from build123d import *

# Parameters (mm, degrees)
PAD002_DEPTH            = 5
SKETCH015_R             = 35
SKETCH015_R_2           = 1.6
POCKET005_DEPTH         = 5.001
SKETCH013_R             = 3.5
SKETCH013_R_2           = 1.7
POCKET004_DEPTH         = 5.001
SKETCH025_W             = 47
SKETCH025_H             = 51
POCKET027_DEPTH         = 2.5
BODY002_PLACEMENT_ANGLE = 180


with BuildPart() as part:
    # Sketch014 → Pad002 (new body)
    with BuildSketch(Plane.XY):
        with BuildLine():
            Line((0, 67.42), (0, -55.65))
            Line((0, -55.65), (-117.94, -55.65))
            ThreePointArc((-127.64, -49.11), (-122.947197, -52.613151), (-117.94, -55.65))
            ThreePointArc((-146.95, -26.77), (-138.520798, -38.999541), (-127.64, -49.11))
            ThreePointArc((-148.54, 6.09), (-150.980867, -10.496574), (-146.95, -26.77))
            ThreePointArc((-134.5, 26.2), (-142.831473, 17.060618), (-148.54, 6.09))
            ThreePointArc((-94.13, 48.54), (-115.023795, 38.650843), (-134.5, 26.2))
            ThreePointArc((0, 67.42), (-48.036997, 62.826084), (-94.13, 48.54))
        make_face()
    extrude(amount=PAD002_DEPTH)

    # Sketch015 (on Face10 of Pad002) → Pocket005 (cut, through all)
    with BuildSketch(Plane.XY.offset(5)):
        with Locations((-90.05, -4.36)):
            Circle(SKETCH015_R)
        with Locations((-119.571708, 25.161708)):
            Circle(SKETCH015_R_2)
        with Locations((-60.528292, 25.161708)):
            Circle(SKETCH015_R_2)
        with Locations((-60.528292, -33.881708)):
            Circle(SKETCH015_R_2)
        with Locations((-119.571708, -33.881708)):
            Circle(SKETCH015_R_2)
    extrude(amount=-POCKET005_DEPTH, mode=Mode.SUBTRACT)

    # Sketch013 (on Face5 of Pocket005) → Pocket004 (cut, through all)
    with BuildSketch(Plane.XY.offset(5)):
        with Locations((-30, -40)):
            Circle(SKETCH013_R)
        with Locations((-43.55, 21.8)):
            Circle(SKETCH013_R_2)
        with Locations((-43.55, -21.8)):
            Circle(SKETCH013_R_2)
        Polygon((0, 25.5), (-38.85, 25.5), (-38.85, 18.5), (-46.75, 18.5), (-46.75, -18.5), (-38.85, -18.5), (-38.85, -25.5), (0, -25.5), align=None)
    extrude(amount=-POCKET004_DEPTH, mode=Mode.SUBTRACT)

    # Sketch025 → Pocket027 (cut)
    with BuildSketch(Plane.XY):
        with Locations((-23.5, 0)):
            Rectangle(SKETCH025_W, SKETCH025_H)
    extrude(amount=POCKET027_DEPTH, mode=Mode.SUBTRACT)


with BuildPart() as part_1:
    # Body002 placement: moved
    add(part.part.moved(Location((0, 0, 2))).rotate(Axis((0, 0, 2), (0, 1, 0)), BODY002_PLACEMENT_ANGLE))


solid = part_1.part
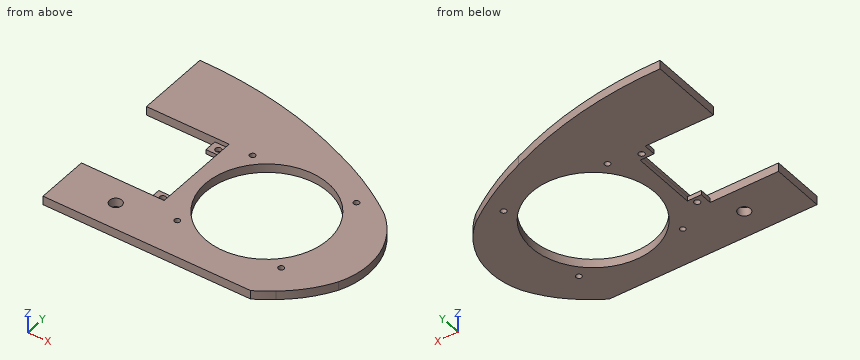
The listing builds one solid part. Answer for the finished solid, in the listing's coordinates (mm). Coordinates: 2 decimals unless noted, no trailing zeros. Order: outer loops, then holes, each group sorted by start corner. A loop starts at its lowest first (then second) coordinate and runs counter-clockwise, first axis right, second up.
Q1. Consider line 1 (X direction, y = 24, z = -1.8); line 2 (Y direction, x = 43.55, z = -1.95); line 3 (X direction, y = 24.5, z = 0.5). Determine where each line is inside the solid, lowest interval first.
Q2. A cutting plane is placed at D-D, the plane z = 0.7. Write down the section's boundary in (x, y).
Q3. Given P1, Ø0.8, axis at y = -11.5, z = 0, coming from the -X side; P2, Ø0.8, axis at y = -21.5, z = -1.5, coming from the -X side; P3, Ø0.8, axis at y = -5, z = -1.5, coming from the -X side, each flat-ended and moving along its own axis, determine where each tip first touches the part or whether it passes through.
Q4. A cutting plane is placed at A-A, the plane x = 90.05. Write down the section's boundary in (y, z).
Q5. A cutting plane is placed at C-C, the plane x = 43.55. Write down the section's boundary in (y, z).
Q6. A cutting plane is placed at B-B, the plane y = 21.8. Write down the section's boundary in (x, z), and give its area (3 significant figures).
Answers follow:
1. line 1: x = 38.85 to 59.43, 61.63 to 69.54, 110.56 to 118.47, 120.67 to 136.93
1. line 2: y = -55.65 to -23.5, -20.1 to -18.5, 18.5 to 20.1, 23.5 to 63.68
1. line 3: x = 47 to 59.07, 61.99 to 70.25, 109.85 to 118.11, 121.03 to 136.4
2. outline: (0, -55.65) - (117.94, -55.65) arc R60.98 ccw to (127.64, -49.11) arc R68.08 ccw to (146.95, -26.77) arc R43.38 ccw to (148.54, 6.09) arc R47.81 ccw to (134.5, 26.2) arc R182.51 ccw to (94.13, 48.54) arc R235.57 ccw to (0, 67.42) - (0, 25.5) - (47, 25.5) - (47, -25.5) - (0, -25.5) - close; hole circle Ø7 at (30, -40); hole circle Ø70 at (90.05, -4.36); hole circle Ø3.2 at (60.53, -33.88); hole circle Ø3.2 at (60.53, 25.16); hole circle Ø3.2 at (119.57, -33.88); hole circle Ø3.2 at (119.57, 25.16)
3. P1: stops at x = 47
3. P2: stops at x = 38.85
3. P3: stops at x = 46.75
4. outline: (-55.65, -3) - (-39.36, -3) - (-39.36, 2) - (-55.65, 2) - close; (30.64, -3) - (50.24, -3) - (50.24, 2) - (30.64, 2) - close
5. outline: (-55.65, -3) - (-23.5, -3) - (-23.5, -0.5) - (-25.5, -0.5) - (-25.5, 2) - (-55.65, 2) - close; (-20.1, -3) - (-18.5, -3) - (-18.5, -0.5) - (-20.1, -0.5) - close; (18.5, -3) - (20.1, -3) - (20.1, -0.5) - (18.5, -0.5) - close; (23.5, -3) - (63.68, -3) - (63.68, 2) - (25.5, 2) - (25.5, -0.5) - (23.5, -0.5) - close
6. outline: (38.85, -3) - (41.85, -3) - (41.85, -0.5) - (38.85, -0.5) - close; (45.25, -3) - (66.8, -3) - (66.8, 2) - (47, 2) - (47, -0.5) - (45.25, -0.5) - close; (113.3, -3) - (139.05, -3) - (139.05, 2) - (113.3, 2) - close
6. area: 240 mm2
